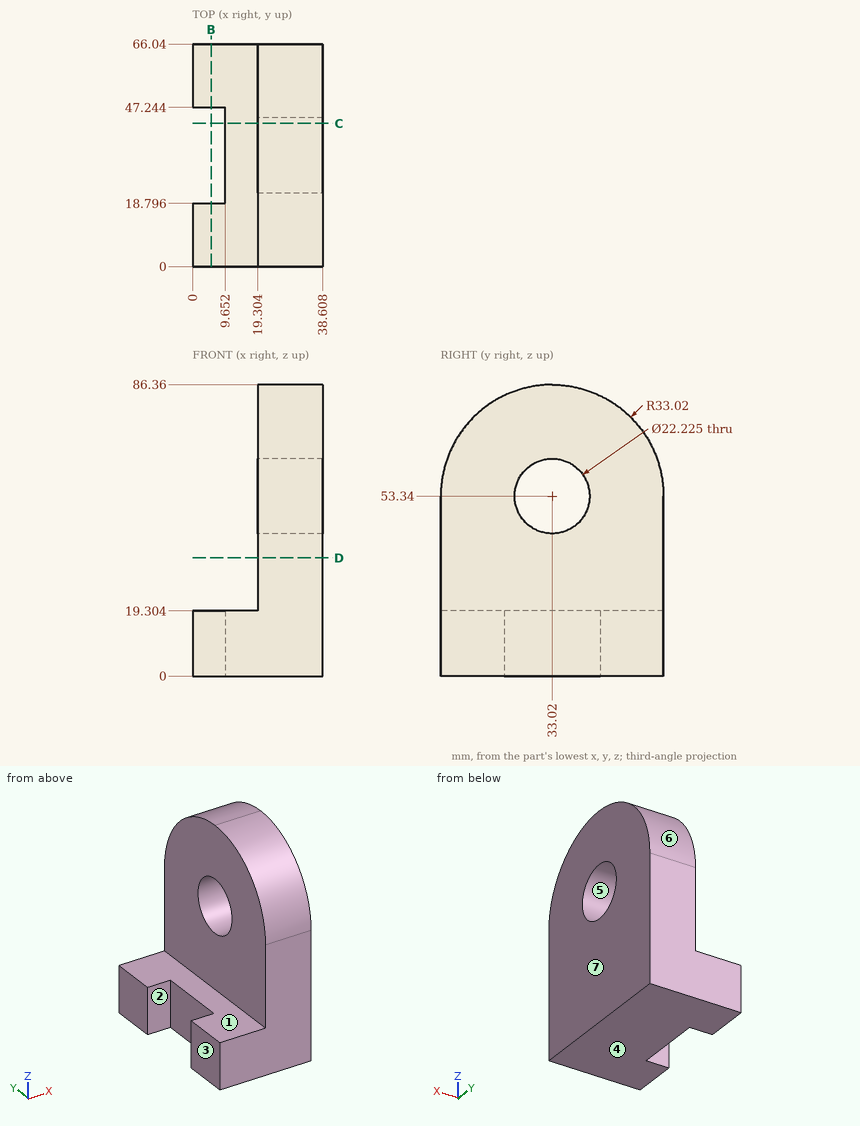
The drawing under review shows one solid part. Ordinate dimensions are in mm from its lowest x, y, z. A direction names the side the tool comes from. Round coordinates to 2 decimals unless told otherwise and drop trailing zeros. Loops run counter-clockwise (first coordinate to the right, second up) from the corner with the lowest first, then second, coordinate; pieces in that order, holes last. Notation, with made-up numbers: (-28, 2.5) -> (-23, 2.5) arc R26 ccw to (-23, 34.5) -> close; hole circle Ø10 at (-4.75, 0). An arc over 180 degrees is marked (long way). Answer in a Markdown table with one row per item.
1) Consider section D-D, the plane z = 35. Write out the cut boundary in (x, y).
Taken from the geometry:
| item | result |
|---|---|
| outline | (19.3, 0) -> (38.61, 0) -> (38.61, 66.04) -> (19.3, 66.04) -> close |
2) For pin 1 Ø8 at (y, z) = (55.5, 74.5) entering from -X; pin 2 Ø21 at (y, z) = (30, 13.5) entering from -X; pin 3 Ø3 at (x, y) = (14.5, 35) entering from +Z, all flat-tipped, find the tip position at first contact; note any pin that passes through.
Taken from the geometry:
| item | result |
|---|---|
| pin 1 | stops at x = 19.3 |
| pin 2 | stops at x = 9.65 |
| pin 3 | stops at z = 19.3 |
3) Consider section C-C, the plane y = 42.5. Write out the cut boundary in (x, z), plus the area to 3 significant figures.
Taken from the geometry:
| item | result |
|---|---|
| outline | (9.65, 0) -> (38.61, 0) -> (38.61, 47.54) -> (19.3, 47.54) -> (19.3, 19.3) -> (9.65, 19.3) -> close; (19.3, 59.14) -> (38.61, 59.14) -> (38.61, 84.97) -> (19.3, 84.97) -> close |
| area | 1,600 mm² |
4) Tool access review of the marked faces 1, 2 and 3: name each direction out of +Z, -Z, +X, -X, +Y, -Y from which nothing blocks a thin tool from reaching the whole face with its end or side.
Taken from the geometry:
| item | result |
|---|---|
| face 1 | +Z, -X, +Y, -Y |
| face 2 | +Z, -Z, -X |
| face 3 | +Z, -Z, -X, +Y, -Y |
5) Draft analysis for pull direction Z (two halves, no side actions). For the marked faces 4, 5, 6 and 7, state which applies: pulls with the +Z half, pulls with the -Z half, needs draft (parallel to the pull), parting line crosses it, or undercut.
Taken from the geometry:
| item | result |
|---|---|
| face 4 | pulls with the -Z half |
| face 5 | undercut |
| face 6 | pulls with the +Z half |
| face 7 | needs draft |
6) Wall thickness on line 1 along Y through (x, z) = (5, 7.5); line 2 along Y through (x, z) = (32, 53); line 3 along X through (y, z) = (15, 25): over which ranges is each line inside the solid? List them lowest first.
Taken from the geometry:
| item | result |
|---|---|
| line 1 | y = 0 to 18.8, 47.24 to 66.04 |
| line 2 | y = 0 to 21.91, 44.13 to 66.04 |
| line 3 | x = 19.3 to 38.61 |
7) Consider section B-B, the plane x = 5.5. Write out the cut boundary in (y, z), plus the area to 3 significant figures.
Taken from the geometry:
| item | result |
|---|---|
| outline | (0, 0) -> (18.8, 0) -> (18.8, 19.3) -> (0, 19.3) -> close; (47.24, 0) -> (66.04, 0) -> (66.04, 19.3) -> (47.24, 19.3) -> close |
| area | 726 mm² |
